from build123d import *

# Parameters (mm, degrees)
SKETCH1_R             = 2.00000108
BOSS_EXTRUDE1_DEPTH   = 41.275
M3_TAPPED_HOLE1_D     = 2.5
M3_TAPPED_HOLE1_DEPTH = 6.35
M3_TAPPED_HOLE1_TIP   = 0.751075774


with BuildPart() as part:
    # Sketch1 → Boss-Extrude1 (new body)
    with BuildSketch(Plane.XY):
        Polygon((2.213234223, 6.990345314), (-4.947199511, 5.411889719), (-7.160433735, -1.578455595), (-2.213234223, -6.990345314), (4.947199511, -5.411889719), (7.160433735, 1.578455595), align=None)
        Circle(SKETCH1_R, mode=Mode.SUBTRACT)
    extrude(amount=BOSS_EXTRUDE1_DEPTH)

    # M3 Tapped Hole1
    with Locations(Plane(origin=(-1.394683733, 6.195011051, 2.448450975), x_dir=(0.976553939578, 0.21527285731, 0), z_dir=(-0.21527285731, 0.976553939578, 0))):
        with Locations((0, 0)):
            Hole(M3_TAPPED_HOLE1_D / 2, depth=M3_TAPPED_HOLE1_DEPTH)
            with Locations((0, 0, -(M3_TAPPED_HOLE1_DEPTH + M3_TAPPED_HOLE1_TIP / 2))):  # 118° drill point
                Cone(0, M3_TAPPED_HOLE1_D / 2, M3_TAPPED_HOLE1_TIP, mode=Mode.SUBTRACT)


solid = part.part
Can you work these out from the model? Positions are in its coordinate system, mm. Coordinates: 2 decimals unless noted, no trailing zeros. Order: outer loops, then holes, each group sorted by start corner. A loop starts at its lowest first (then second) coordinate and runs counter-clockwise, first axis right, second up. Notation, with made-up numbers: M 65,-10 L 123,-10 A18 ccw 123,20 Z; hole C -33.75,11 d5. An arc over 180 degrees is marked long. Write item = value, one per line.
(1) I need wall thicknesses on line 1 along Y through (x, z) = (0, 22.5); line 2 along Y through (x, z) = (0.5, 23); line 3 along Y through (x, z) = (-4.25, 35). Which ranges of each line are inside material? Lowest first, please. Write a range as [from, to].
Results are:
line_1 = [-6.5, -2], [2, 6.5]
line_2 = [-6.39, -1.94], [1.94, 6.61]
line_3 = [-4.76, 5.57]
(2) Suppose I cut it at C-C on y = -3.25. Please give me the cut outline in (x, z) (3 decimals), plus the area to 3 significant figures.
Results are:
outline = M -5.632,0 L 5.632,0 L 5.632,41.275 L -5.632,41.275 Z
area = 465 mm2
(3) Suppose I cut it at B-B on z = 31. Please give me the cut outline in (x, y).
Results are:
outline = M -7.16,-1.58 L -2.21,-6.99 L 4.95,-5.41 L 7.16,1.58 L 2.21,6.99 L -4.95,5.41 Z; hole C 0,0 d4
(4) Suppose I cut it at A-A on y = 0.5. Please give me the cut outline in (x, z) (1 decimal).
Results are:
outline = M -6.5,0 L -1.9,0 L -1.9,41.3 L -6.5,41.3 Z; M 1.9,0 L 6.8,0 L 6.8,41.3 L 1.9,41.3 Z
(5) If we mould it in two halves opening along X, with no side actions, what happens to faces 1 (the face through (-6.038, 1.966, 20.349)), 2 (the face through (-0.605, 3.871, 3.669)), 3 (the face through (1.32, -6.21, 20.35))? For each: pulls with the +X half, pulls with the -X half, needs draft (parallel to the pull), parting line crosses it, or undercut.
Results are:
face_1 = pulls with the -X half
face_2 = undercut
face_3 = pulls with the +X half
(6) For pin 1 Ø1.5 at (y, z) = (3.5, 30) entering from +X; pin 2 Ø3 at (x, z) = (1, 4.5) entering from +Y; pin 3 Ø3 at (x, y) = (0, 0) entering from -Z; pin 4 Ø4 at (y, z) = (5, 10.5) entering from -X, each with a flat end and sliding along its axis, tell me the tip position at first contact or that it passes through.
Results are:
pin_1 = 6.09
pin_2 = 6.99
pin_3 = through
pin_4 = -5.71
